For this review, take the finished solid that the model builds, in its own axes (mm). Round coordinates to 2 decimals unless told otherwise and drop trailing zeros. Write each loop counter-clockwise with the first axis right and the second up, starting at its lowest first coordinate (ties: lowest second). Pieces come first, ordered by that corner, then holes. Notation, with made-up numbers: (22, 55) - (77, 55) arc R13 cw to (77, 63) - close; hole circle Ø10 at (23, 84.5). An arc over 180 degrees is marked (long way). Answer in a Markdown table with one row per item. Add a question column.
Autodesk Inventor part; units mm, degrees
ref_plane "YZ Plane" through (0, 0, 0) normal (1, 0, 0) x (0, 1, 0)
ref_plane "XZ Plane" through (0, 0, 0) normal (0, 1, 0) x (-1, 0, 0)
ref_plane "XY Plane" through (0, 0, 0) normal (0, 0, 1) x (1, 0, 0)
sketch "Sketch1" plane through (0, 0, 0) normal (0, 0, 1) x (1, 0, 0)
  line L0 (-7, -40) -> (7, -40)
  line L1 (7, -40) -> (7, 40)
  line L2 (7, 40) -> (-7, 40)
  line L3 (-7, 40) -> (-7, -40)
  line L4 (-7, -40) -> (7, 40) construction
  line L5 (7, -40) -> (-7, 40) construction
  point P0 (0, 0)
  dimension "d0" = 14
  dimension "d1" = 80
extrude "Extrusion1" add sketch "Sketch1" along normal blind 10
chamfer "Chamfer1" distance 5 distance2 8 1 edges at (0, -40, 10) measured on face at (-2.3333, 13.3333, 10)
chamfer "Chamfer2" distance 2 angle 45 3 edges at (7, 2.5, 10) (-7, 2.5, 10) (0, -35, 10)
equation "\"d0\" = 2 * blackkey_halfwidth"
equation "\"d1\" = blackkey_length"
equation "\"d2\" = 0.5 * key_height"
properties part number "key_black"
Q1. Add section C-C on z = 4. State the section outline as (x, y) points.
Q2. Insertion check: pin 1 Ø5 at (x, z) = (2.5, 6.5) entering from -Y. The pin has a flat end and moves straight along its axis. Give the tip position at first contact, or say it passes through.
Q3. To check wall thickness, follow probe 1 along Y at (x, z) = (-4.5, 9); probe 2 along Y at (x, z) = (2.5, 3) (3 decimals); probe 3 along X at (y, z) = (-24, 8.25). State the ranges of each line that lie inside material, in increasing order.
Q4. Add section A-A on x = 3. State the section outline as (y, z) points, then the cut area to 3 significant figures.
Q5. Add section B-B on y = -21.5. State the section outline as (x, z) points.
Answer sheet:
| question | item | result |
|---|---|---|
| 1 | outline | (-7, -38.75) - (7, -38.75) - (7, 40) - (-7, 40) - close |
| 2 | pin 1 | stops at y = -38.75 |
| 3 | probe 1 | y = -34.8 to 40 |
| 3 | probe 2 | y = -39.375 to 40 |
| 3 | probe 3 | x = -6.75 to 6.75 |
| 4 | outline | (-40, 0) - (40, 0) - (40, 10) - (-33, 10) - (-36.06, 8.3) - (-40, 2) - close |
| 4 | area | 778 mm² |
| 5 | outline | (-7, 0) - (7, 0) - (7, 8) - (5, 10) - (-5, 10) - (-7, 8) - close |
